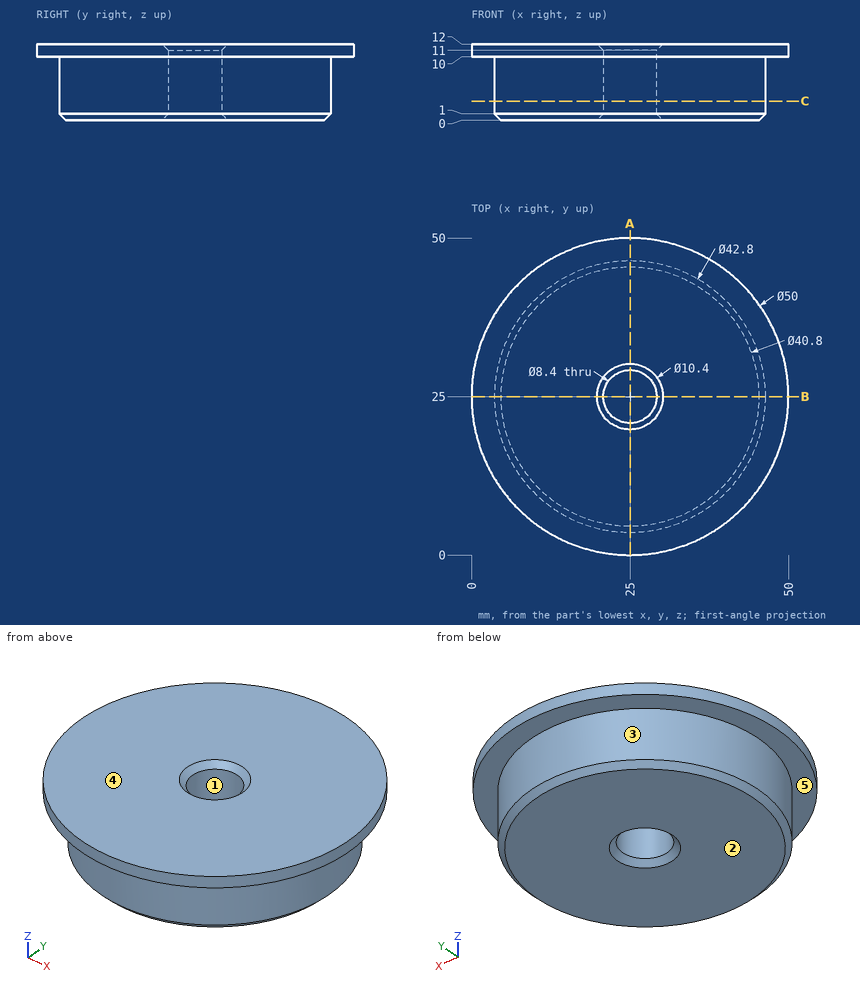
Study the drawing (mm; zero at the part's minimum x, y, z) and answer. A direction names the side the tool comes from. Coordinates: 2 decimals unless noted, no trailing zeros. Loops run counter-clockwise (first coordinate to the right, second up) from the corner with the lowest first, then second, coordinate; pieces in that order, holes last. Notation, with made-up numbers: M -17,43.5 L -11,43.5 A13 ccw -11,58.5 Z; hole C 18.25,38.5 d6. An arc over 180 degrees is marked long. Answer in a Markdown table with one row per item. Add a question column.
1. Flat-ended cylindrical pins translate along their axes: P1, Ø4, axis at x = 20.5, z = 10.5, coming from the -Y side; P2, Ø2, axis at x = 8.5, y = 7.5, coming from the -Z side; P3, Ø1.5, axis at y = 35, z = 4, coming from the +X side; P4, Ø6.5, axis at x = 25, y = 25, coming from the -Z side. Find the tip coordinate at first contact, or state that the pin passes through.
2. The mould has two halves that part along X. Classify the marked faces 1, 2 and 3: pulls with the +X half, pulls with the -X half, needs draft (parallel to the pull), parting line crosses it, or undercut.
3. A tool of negligible diameter and unlimited length cuts with its end or side. For the marked faces 4 and 5, from which of +Z, -Z, +X, -X, +Y, -Y can it reach the whole face along a straight path? Write none if from no direction.
4. Find section A-A, the plane x = 25. Write down the section's boundary in (y, z), then the cut area to 3 significant figures.
5. Consider L1, parallel to Y at x = 25, z = 8.5; L2, parallel to Z at x = 3, y = 28.5; L3, parallel to X at y = 24, z = 9.5. Determine where each line is inside the solid, lowest interval first.
6. Find section C-C, the plane z = 3. Write down the section's boundary in (x, y), then the cut area to 3 significant figures.
Reported:
| question | item | result |
|---|---|---|
| 1 | P1 | stops at y = 0.13 |
| 1 | P2 | stops at z = 10 |
| 1 | P3 | stops at x = 44.3 |
| 1 | P4 | passes through |
| 2 | face 1 | undercut |
| 2 | face 2 | needs draft |
| 2 | face 3 | parting line crosses it |
| 3 | face 4 | +Z, +X, -X, +Y, -Y |
| 3 | face 5 | -Z |
| 4 | outline | M 0,10 L 3.6,10 L 3.6,1 L 4.6,0 L 19.8,0 L 20.8,1 L 20.8,11 L 19.8,12 L 0,12 Z; M 29.2,1 L 30.2,0 L 45.4,0 L 46.4,1 L 46.4,10 L 50,10 L 50,12 L 30.2,12 L 29.2,11 Z |
| 4 | area | 424 mm^2 |
| 5 | L1 | y = 3.6 to 20.8, 29.2 to 46.4 |
| 5 | L2 | z = 10 to 12 |
| 5 | L3 | x = 3.62 to 20.92, 29.08 to 46.38 |
| 6 | outline | C 25,25 d42.8; hole C 25,25 d8.4 |
| 6 | area | 1,380 mm^2 |
